```python
from build123d import *

# Parameters (mm, degrees)
BOSS_EXTRUDE1_DEPTH = 215
SHELL1_START        = 4
SHELL1_DEPTH        = 207
SKETCH3_R           = 2.1
CUT_EXTRUDE1_DEPTH  = 231.683632934
FILLET1_R           = 2


# Read off the part's stored shape, not the designer's step: Shell1
with BuildPart() as part:
    # Sketch1 → Boss-Extrude1 (new body)
    with BuildSketch(Plane(origin=(0, 0, 0), x_dir=(0, 0, -1), z_dir=(1, 0, 0))):
        with BuildLine():
            Line((70.261974321, -14.858488677), (65.445567386, -14.858488677))
            ThreePointArc((65.445567386, -14.858488677), (64.047743646, -14.288904278), (63.446098501, -12.904577468))
            Line((63.446098501, -12.904577468), (62.535908701, 26.582164322))
            ThreePointArc((62.535908701, 26.582164322), (63.05617043, 27.974338618), (64.393258315, 28.623197251))
            Line((64.393258315, 28.623197251), (75.379560776, 29.405858418))
            ThreePointArc((75.379560776, 29.405858418), (76.868805698, 28.889174231), (77.521211792, 27.454190163))
            Line((77.521211792, 27.454190163), (78.259876122, -6.675276303))
            ThreePointArc((78.259876122, -6.675276303), (75.98323725, -12.450192398), (70.261974321, -14.858488677))
        make_face()
    extrude(amount=BOSS_EXTRUDE1_DEPTH)

    # Shell1 outline → Shell1 (cut)
    with BuildSketch(Plane.YZ.offset(SHELL1_START)):
        with BuildLine():
            Line((-10.858488677, -63.398935097), (-10.858488677, -70.261974321))
            ThreePointArc((-10.858488677, -70.261974321), (-9.652532179, -73.124372077), (-6.761828222, -74.260806245))
            Line((-6.761828222, -74.260806245), (25.266638922, -73.567620252))
            Line((25.266638922, -73.567620252), (24.484187937, -62.584268141))
            Line((24.484187937, -62.584268141), (-10.858488677, -63.398935097))
        make_face()
    extrude(amount=SHELL1_DEPTH, mode=Mode.SUBTRACT)

    # Sketch3 → Cut-Extrude1 (cut, through all)
    with BuildSketch(Plane(origin=(215, 0, 0), x_dir=(0, 0, -1), z_dir=(1, 0, 0))):
        with Locations((70.261974321, -6.858488677)):
            Circle(SKETCH3_R)
        with Locations((69.886409545, 21.014527834)):
            Circle(SKETCH3_R)
    extrude(amount=-CUT_EXTRUDE1_DEPTH, mode=Mode.SUBTRACT)

    # Fillet1
    fillet1_edges = [part.edges().sort_by_distance(p)[0] for p in [
        (107.5, 25.266638922, -73.567620252),
    ]]
    fillet(fillet1_edges, radius=FILLET1_R)


solid = part.part
```
The listing builds one solid part. Answer for the finished solid, in the listing's coordinates (mm). A direction names the side the tool comes from. Coordinates: 2 decimals unless noted, no trailing zeros. Write each loop counter-clockwise with the first axis right and the second up, starting at its lowest first coordinate (ties: lowest second). Pieces come first, ordered by that corner, then holes. Notation, with made-up numbers: M 7,-9 L 23,-9 A28 ccw 23,21 Z; hole C -20.5,28 d4. An arc over 180 degrees is marked long. Use a Markdown table: item, result. Add a question column.
1. For a pull along Y with two mould halves and no side action, classify faces 4 (the flat face through (4, 7, -68)), 5 (the flat face through (0, 8, -71)), 6 (the flat face through (106, 29.01, -69.81)) as +Y half, -Y half, draft (parallel to the pull), parting line (faces both ways), or undercut.
2. Section B-B (y = 12.5) is taken. Give the vertices of the cut face in (x, z), plus the area to 3 significant figures.
3. Section A-A (x = 75.5) is taken. Give the vertices of the cut face in (y, z).
4. Straight lines are drawn through the part: line 1 along X through (y, z) = (11, -69); line 2 along Y through (x, z) = (145, -68.25); line 3 along Y through (x, z) = (201, -69). For each, find the intervals that lie inside material, in ascending order. Write a range as [from, to].
5. Which of the six approach directions +Z, -Z, +X, -X, +Y, -Y give full straight-line access (tool end or side, diameter ignored) to faces 1 (the flat face through (106, -10.858, -67)), 2 (the flat face through (106.051, 24.805, -67.09)), 3 (the flat face through (106, -14.858, -68))?
6. Given P1, Ø2, axis at x = 32, z = -70.5, coming from the +Y side; P2, Ø2, axis at x = 56.5, z = -66, coming from the +Y side; P3, Ø3, axis at x = 133, y = -8, coming from the +Z side, each flat-ended and moving along its own axis, determine where each tip first touches the part or whether it passes through.
7. Section C-C (y = 3.5) is taken. Give the vertices of the cut face in (x, z), plus the area to 3 significant figures.
Data:
| question | item | result |
|---|---|---|
| 1 | face 4 | undercut |
| 1 | face 5 | draft |
| 1 | face 6 | +Y half |
| 2 | outline | M 0,-77.84 L 215,-77.84 L 215,-62.86 L 211,-62.86 L 211,-73.84 L 4,-73.84 L 4,-62.86 L 0,-62.86 Z |
| 2 | area | 948 mm2 |
| 3 | outline | M -14.86,-70.26 A8 ccw -6.68,-78.26 L 27.45,-77.52 A2 ccw 29.41,-75.38 L 28.62,-64.39 A2 ccw 26.58,-62.54 L 24.48,-62.58 L 25.12,-71.47 A2 cw 23.17,-73.61 L -6.76,-74.26 A4 cw -10.86,-70.26 L -10.86,-63.4 L -12.9,-63.45 A2 ccw -14.86,-65.45 Z |
| 4 | line 1 | x = [0, 4], [211, 215] |
| 4 | line 2 | y = [-14.86, -10.86], [24.89, 28.9] |
| 4 | line 3 | y = [-14.86, -10.86], [24.94, 28.95] |
| 5 | face 1 | +Z |
| 5 | face 2 | none |
| 5 | face 3 | +Z, -Z, +X, -X, -Y |
| 6 | P1 | stops at y = 29.13 |
| 6 | P2 | stops at y = 28.81 |
| 6 | P3 | stops at z = -73.27 |
| 7 | outline | M 0,-78.04 L 215,-78.04 L 215,-63.07 L 211,-63.07 L 211,-74.04 L 4,-74.04 L 4,-63.07 L 0,-63.07 Z |
| 7 | area | 948 mm2 |
